Part model, mm, in its own coordinate system. A direction names the side the tool comes from. Round coordinates to 2 decimals unless told otherwise and drop trailing zeros. Loops run counter-clockwise (first coordinate to the right, second up) from the corner with the lowest first, then second, coordinate; pieces in that order, holes last.
1) Band-saw the part on D-D, the plane x = -32. Write the cut outline in (y, z), then the cut area to 3 significant figures.
2) 3-axis set-ups, long thin cutter, end or side, ignore diameter. For faces 5 (the flat face through (-2, 24, 25)), 6 (the flat face through (-30, 4, 25)): which of +Z, -Z, +X, -X, +Y, -Y reach the whole face in a straight line?
3) Band-saw the part on C-C, the plane z = 35. Write the cut outline in (x, y), then the cut area to 3 significant figures.
4) Band-saw the part on A-A, the plane z = 25. Write the cut outline in (x, y).
5) Probe line 1 (Z direction, x = -21.5, y = 2.7); line 2 (Z direction, x = -1.15, y = 16); line 3 (Z direction, x = -23, y = 1.5). List the from-to ranges inside material, lowest first.
6) Mould opens along Y. For faces 1 (the flat face through (-3.6, 15, 25)), 2 (the cylindrical face through (-11.84, 2.92, 49.92)), 3 (the cylindrical face through (-2, 16, 17)), 4 (the flat face through (-16, 0, 25)) say: +Y half, -Y half, draft (parallel to the pull), parting line (faces both ways), or undercut.
7) Band-saw the part on B-B, the plane y = 16. Write the cut outline in (x, z).
8) Drop flat-ended pins along their axis: P1, Ø10, axis at x = -19.5, z = 42, coming from the -Y side; P2, Ø6, axis at x = -18.5, y = 5, coming from the +Z side; P3, Ø2.5, axis at y = 16, z = 35, coming from the -X side; P4, Ø6, axis at y = 18, z = 18.5, coming from the -X side. Give the stop position or say it passes through.
from build123d import *

# Parameters (mm, degrees)
PAD003_DEPTH    = 50
SKETCH_R        = 2.6
SKETCH_R_2      = 4.7
POCKET_DEPTH    = 4
SKETCH005_R     = 2
POCKET001_DEPTH = 3.6
CHAMFER_SIZE    = 5
FILLET_R        = 23


with BuildPart() as part:
    # Sketch003 → Pad003 (new body)
    with BuildSketch(Plane.XY):
        Polygon((-43, 4), (-3.6, 4), (-3.6, 24), (0, 24), (0, 0), (-43, 0), align=None)
    extrude(amount=PAD003_DEPTH)

    # Sketch → Pocket (cut)
    with BuildSketch(Plane.XZ):
        with Locations((-21.5, 43.25)):
            Circle(SKETCH_R)
        with Locations((-21.5, 6.75)):
            Circle(SKETCH_R)
        with Locations((-21.5, 25)):
            Circle(SKETCH_R_2)
    extrude(amount=-POCKET_DEPTH, mode=Mode.SUBTRACT)

    # Sketch005 → Pocket001 (cut)
    with BuildSketch(Plane.YZ):
        with Locations((16, 35)):
            Circle(SKETCH005_R)
        with Locations((16, 15)):
            Circle(SKETCH005_R)
    extrude(amount=-POCKET001_DEPTH, mode=Mode.SUBTRACT)

    # Chamfer
    chamfer_edges = [part.edges().sort_by_distance(p)[0] for p in [
        (-3.6, 4, 25),
    ]]
    chamfer(chamfer_edges, length=CHAMFER_SIZE)

    # Fillet
    fillet_edges = [part.edges().sort_by_distance(p)[0] for p in [
        (-1.8, 24, 0),
        (-1.8, 24, 50),
    ]]
    fillet(fillet_edges, radius=FILLET_R)


solid = part.part
Reported:
1. outline: (0, 0) - (1, 0) arc R23 ccw to (4, 0.2) - (4, 49.8) arc R23 ccw to (1, 50) - (0, 50) - close
1. area: 200 mm2
2. face 5: +Z, -Z, +X, -X, +Y
2. face 6: +Z, -Z, -X, +Y
3. outline: (-43, 0) - (0, 0) - (0, 14) - (-3.6, 14) - (-3.6, 9) - (-8.6, 4) - (-43, 4) - close; (-3.6, 18) - (0, 18) - (0, 22.56) - (-3.6, 22.56) - close
3. area: 237 mm2
4. outline: (-43, 0) - (-26.2, 0) - (-26.2, 4) - (-43, 4) - close; (-16.8, 0) - (0, 0) - (0, 24) - (-3.6, 24) - (-3.6, 9) - (-8.6, 4) - (-16.8, 4) - close
5. line 1: z = 0.06 to 4.15, 9.35 to 20.3, 29.7 to 40.65, 45.85 to 49.94
5. line 2: z = 5.56 to 13, 17 to 33, 37 to 44.44
5. line 3: z = 0.01 to 4.63, 8.87 to 20.55, 29.45 to 41.13, 45.37 to 49.99
6. face 1: draft
6. face 2: +Y half
6. face 3: undercut
6. face 4: -Y half
7. outline: (-3.6, 5.56) - (0, 5.56) - (0, 13) - (-3.6, 13) - close; (-3.6, 17) - (0, 17) - (0, 33) - (-3.6, 33) - close; (-3.6, 37) - (0, 37) - (0, 44.44) - (-3.6, 44.44) - close
8. P1: stops at y = 0
8. P2: stops at z = 49.98
8. P3: passes through
8. P4: stops at x = -3.6
